The drawing under review shows one solid part. Ordinate dimensions are in mm from its lowest x, y, z. A direction names the side the tool comes from. Round coordinates to 2 decimals unless told otherwise and drop trailing zeros. Order: outer loops, then holes, each group sorted by start corner. A loop starts at its lowest first (then second) coordinate and runs counter-clockwise, first axis right, second up. Notation, with made-up numbers: (65, 78.5) -> (78, 78.5) arc R14 cw to (78, 104.5) -> close; hole circle Ø4 at (69.5, -18). An arc over 180 degrees is marked (long way). Use a Markdown table: item, result. Add a question column.
1) Consider section B-B (x = 10). State the section outline as (y, z) points.
2) Consider section A-A (z = 10). State the section outline as (x, y) points, plus the area to 3 significant figures.
3) Consider section C-C (y = 4.2). State the section outline as (x, z) points, plus the area to 3 significant figures.
4) Machinability: for the marked faces 3, 4 and 5, which of the approach directions +Z, -Z, +X, -X, +Y, -Y give a long, thin tool a straight path to every point of the face, cutting with its end or side? Answer none if there is none.
5) Clearance check with flat-ended pins moving along their axes: P1, Ø13.5, axis at x = 5, z = 81.5, coming from the +Y side; P2, Ø0.6, axis at y = 3.5, z = 75.5, coming from the +X side. State where each tip first meets the part, or that it passes through.
6) Draft analysis for pull direction Z (two halves, no side actions). For the marked faces 1 and 2, state which applies: pulls with the +Z half, pulls with the -Z half, needs draft (parallel to the pull), parting line crosses it, or undercut.
7) Wall thickness on line 1 along Z through (x, y) = (85, 3.55); line 2 along X through (y, z) = (2.75, 10); line 3 along Y through (x, z) = (13, 84): over which ranges is each line inside the solid? List them lowest first. Write a range as [from, to].
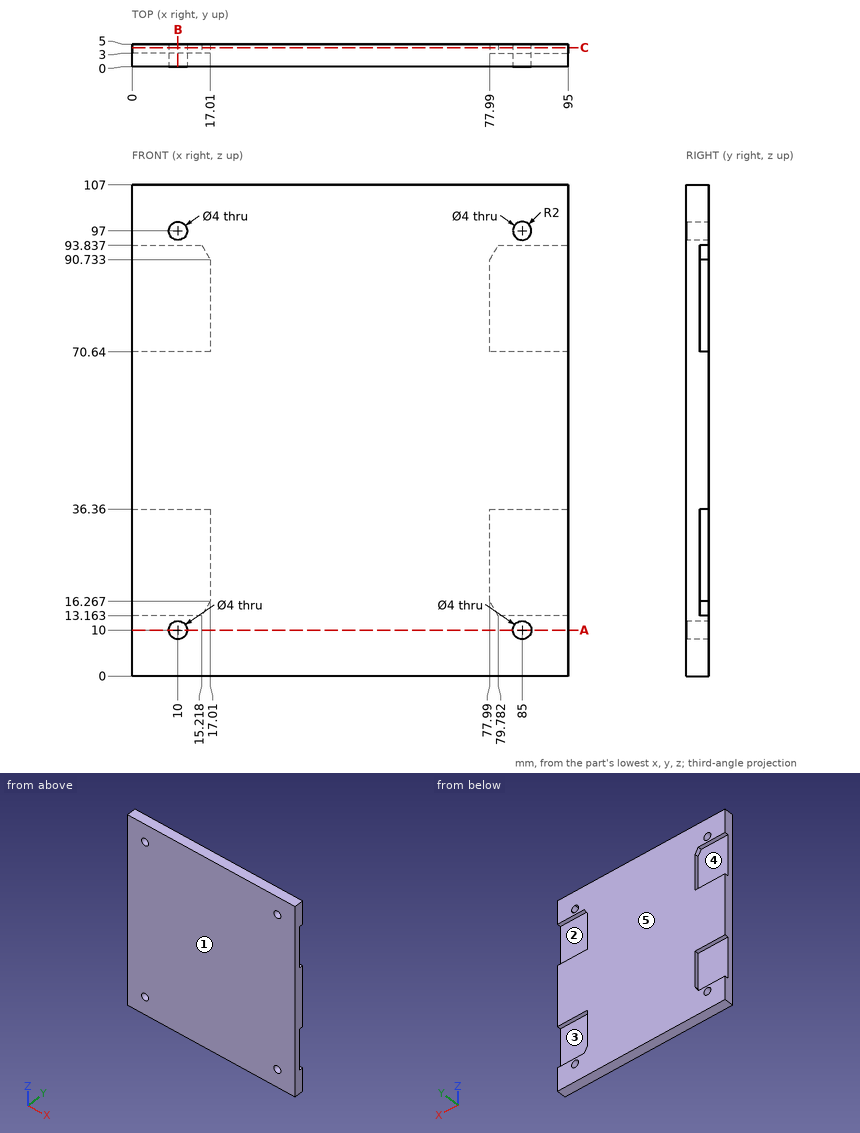
Results list:
| question | item | result |
|---|---|---|
| 1 | outline | (0, 0) -> (5, 0) -> (5, 8) -> (0, 8) -> close; (0, 12) -> (5, 12) -> (5, 13.16) -> (3, 13.16) -> (3, 36.36) -> (5, 36.36) -> (5, 70.64) -> (3, 70.64) -> (3, 93.84) -> (5, 93.84) -> (5, 95) -> (0, 95) -> close; (0, 99) -> (5, 99) -> (5, 107) -> (0, 107) -> close |
| 2 | outline | (0, 0) -> (8, 0) -> (8, 5) -> (0, 5) -> close; (12, 0) -> (83, 0) -> (83, 5) -> (12, 5) -> close; (87, 0) -> (95, 0) -> (95, 5) -> (87, 5) -> close |
| 2 | area | 435 mm2 |
| 3 | outline | (0, 0) -> (95, 0) -> (95, 13.16) -> (79.78, 13.16) -> (77.99, 16.27) -> (77.99, 36.36) -> (95, 36.36) -> (95, 70.64) -> (77.99, 70.64) -> (77.99, 90.73) -> (79.78, 93.84) -> (95, 93.84) -> (95, 107) -> (0, 107) -> (0, 93.84) -> (15.22, 93.84) -> (17.01, 90.73) -> (17.01, 70.64) -> (0, 70.64) -> (0, 36.36) -> (17.01, 36.36) -> (17.01, 16.27) -> (15.22, 13.16) -> (0, 13.16) -> close; hole circle Ø4 at (10, 10); hole circle Ø4 at (10, 97); hole circle Ø4 at (85, 10); hole circle Ø4 at (85, 97) |
| 3 | area | 8,550 mm2 |
| 4 | face 3 | +X, +Y |
| 4 | face 4 | -X, +Y |
| 4 | face 5 | +Z, -Z, +X, -X, +Y |
| 5 | P1 | y = 3 |
| 5 | P2 | x = 77.99 |
| 6 | face 1 | needs draft |
| 6 | face 2 | undercut |
| 7 | line 1 | [0, 8], [12, 13.16], [36.36, 70.64], [93.84, 95], [99, 107] |
| 7 | line 2 | [0, 8], [12, 83], [87, 95] |
| 7 | line 3 | [0, 3] |
